from build123d import *

# Parameters (mm, degrees)
F0_R     = 11.22
F0_R_2   = 9.92
F1_DEPTH = 4
F4_DEPTH = 0.3


with BuildPart() as f1:
    # F0 (on Top) → F1 (new body)
    with BuildSketch(Plane.XY):
        Circle(F0_R)
        Circle(F0_R_2, mode=Mode.SUBTRACT)
    extrude(amount=F1_DEPTH)

    # F3 (on offset) → F4 (cut)
    with BuildSketch(Plane.XZ.offset(11.3)):
        Polygon((0, 3.75), (-2.020726, 0.25), (2.020726, 0.25), align=None)
        with BuildLine():
            Line((-0.1, 0.45), (-1.674316, 0.45))
            Line((-1.674316, 0.45), (-0.9065, 1.779896))
            Line((-0.9065, 1.779896), (-0.89784, 1.774896))
            ThreePointArc((-0.89784, 1.774896), (-0.827242, 0.916552), (-0.1, 0.455186))
            Line((-0.1, 0.455186), (-0.1, 0.45))
        make_face(mode=Mode.SUBTRACT)
        with BuildLine():
            ThreePointArc((-0.1, 0.65655), (-0.766667, 1.416667), (-0.1, 2.176784))
            Line((-0.1, 2.176784), (-0.1, 0.65655))
        make_face(mode=Mode.SUBTRACT)
        with BuildLine():
            Line((0.9065, 1.779896), (1.674316, 0.45))
            Line((1.674316, 0.45), (0.1, 0.45))
            Line((0.1, 0.45), (0.1, 0.455186))
            ThreePointArc((0.1, 0.455186), (0.827242, 0.916552), (0.89784, 1.774896))
            Line((0.89784, 1.774896), (0.9065, 1.779896))
        make_face(mode=Mode.SUBTRACT)
        with BuildLine():
            ThreePointArc((0.1, 2.176784), (0.766667, 1.416667), (0.1, 0.65655))
            Line((0.1, 0.65655), (0.1, 2.176784))
        make_face(mode=Mode.SUBTRACT)
        with BuildLine():
            Line((-0.767816, 2.020104), (-0.1, 3.176795))
            Line((-0.1, 3.176795), (-0.1, 2.378147))
            ThreePointArc((-0.1, 2.378147), (-0.466355, 2.2634), (-0.759155, 2.015104))
            Line((-0.759155, 2.015104), (-0.767816, 2.020104))
        make_face(mode=Mode.SUBTRACT)
        with BuildLine():
            Line((0.1, 2.378147), (0.1, 3.176795))
            Line((0.1, 3.176795), (0.767816, 2.020104))
            Line((0.767816, 2.020104), (0.759155, 2.015104))
            ThreePointArc((0.759155, 2.015104), (0.466355, 2.2634), (0.1, 2.378147))
        make_face(mode=Mode.SUBTRACT)
    extrude(amount=-F4_DEPTH, mode=Mode.SUBTRACT)


solid = f1.part
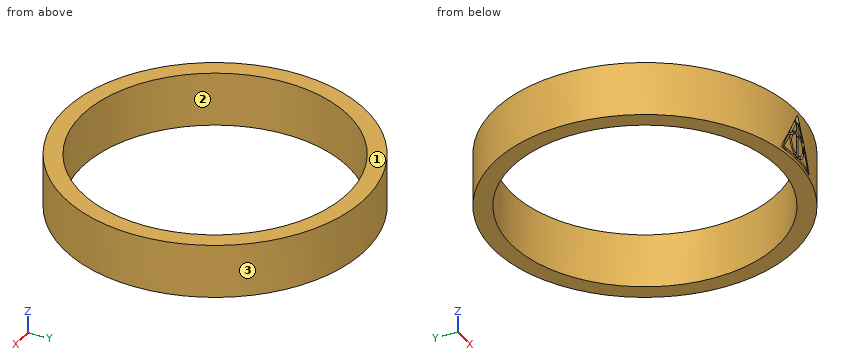
The model under review builds one solid part; all positions refer to its coordinate system, in mm. Face numbers are marked on the shaded views. Give positions to 0.01 mm unless a question says otherwise; leave off trailing zeros. Loops run counter-clockwise (first coordinate to the right, second up) from the corner with the lowest first, then second, coordinate; pieces in that order, holes last. Notation, with made-up numbers: (-28, 6.25) -> (5, 6.25) arc R16 ccw to (5, 30.25) -> close; hole circle Ø1 at (-27, 15.25). An arc over 180 degrees is marked (long way). Put each result on its own line as item: value. Start each with the question number.
1. Wall thickness on probe 1 along Y at (x, z) = (0, 1.45); probe 2 along Y at (x, z) = (-2.75, 2.9); probe 3 along X at (y, z) = (8, 1.4): over which ranges is each line inside the solid? List them lowest first.
2. Clearance check with flat-ended pins moving along their axes: P1, Ø1.5, axis at y = -5.5, z = 3, coming from the +X side; P2, Ø10, axis at x = -2.5, y = -3.5, coming from the +Z side; P3, Ø1, axis at x = 2.5, z = 3.5, coming from the +Y side. State where each tip first meets the part, or that it passes through.
3. We need section B-B on x = -6.5. State the section outline as (y, z) points.
4. Mouldability with a two-part tool opening along Y and no side actions: class the marked faces 1, 2 and 3 as released by +Y, released by -Y, zero draft, split by the parting line, or undercut.
5. We need section C-C on z = 1.15. State the section outline as (x, y) points, then the cut area to 3 significant figures.
6. We need section A-A on y = 0. State the section outline as (x, z) points.
Determined:
1. probe 1: -11 to -9.92, 9.92 to 11.22
1. probe 2: -10.88 to -9.53, 9.53 to 10.88
1. probe 3: -7.87 to -5.87, 5.87 to 7.87
2. P1: x = 10.16
2. P2: through
2. P3: y = 11.04
3. outline: (-9.15, 0) -> (-7.49, 0) -> (-7.49, 4) -> (-9.15, 4) -> close; (7.49, 0) -> (9.15, 0) -> (9.15, 4) -> (7.49, 4) -> close
4. face 1: zero draft
4. face 2: undercut
4. face 3: split by the parting line
5. outline: (-1.5, -11.12) -> (-1.5, -11) -> (-1.27, -11) -> (-1.27, -11.15) arc R11.22 ccw to (-0.93, -11.18) -> (-0.93, -11) -> (-0.72, -11) -> (-0.72, -11.2) arc R11.22 ccw to (-0.1, -11.22) -> (-0.1, -11) -> (0.1, -11) -> (0.1, -11.22) arc R11.22 ccw to (0.72, -11.2) -> (0.72, -11) -> (0.93, -11) -> (0.93, -11.18) arc R11.22 ccw to (1.27, -11.15) -> (1.27, -11) -> (1.5, -11) -> (1.5, -11.12) arc R11.22 ccw (long way) to start; hole circle Ø19.84 at (0, 0)
5. area: 86.2 mm^2
6. outline: (-11.22, 0) -> (-9.92, 0) -> (-9.92, 4) -> (-11.22, 4) -> close; (9.92, 0) -> (11.22, 0) -> (11.22, 4) -> (9.92, 4) -> close
